Job drawing, mm, ordinate dimensions from the low corner. One solid piece. A direction names the side the tool comes from. Round coordinates to 2 decimals unless told otherwise and drop trailing zeros. Loops run counter-clockwise (first coordinate to the right, second up) from the corner with the lowest first, then second, coordinate; pieces in that order, holes last.
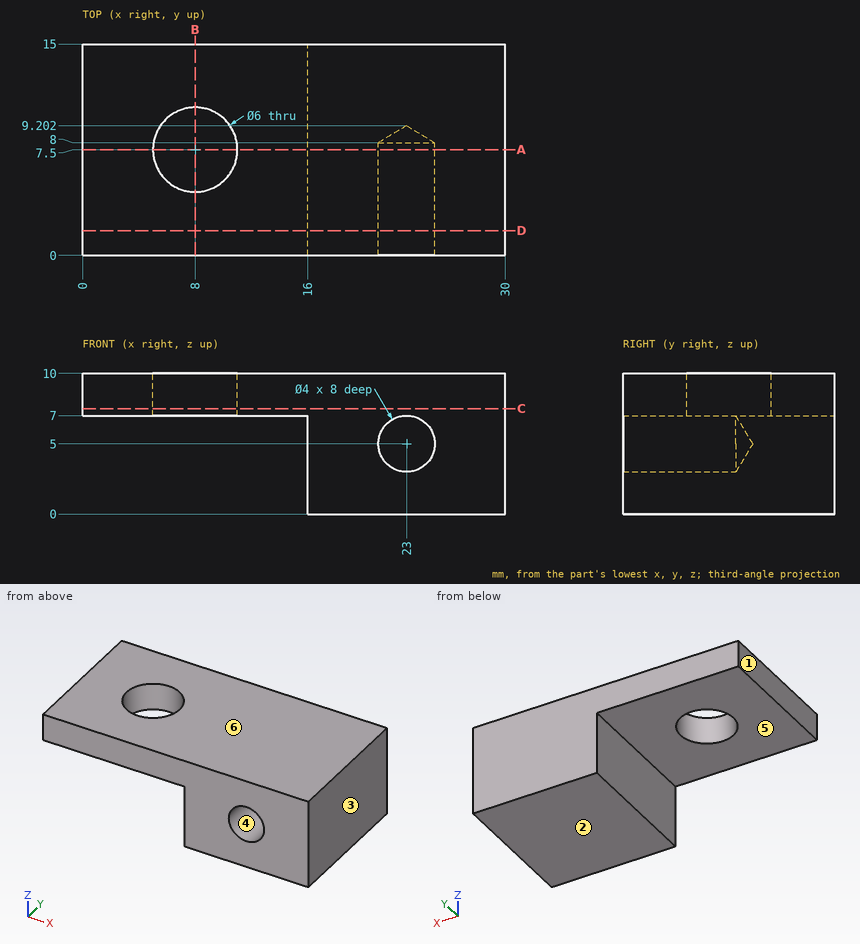
(1) Probe line 1 (Y direction, x = 8, z = 8.1); line 2 (Z direction, x = 23, y = 5.75); line 3 (X direction, y = 6, z = 5). List the from-to ranges inside material, lowest first.
Responses:
line 1: y = 0 to 4.5, 10.5 to 15
line 2: z = 0 to 3, 7 to 10
line 3: x = 16 to 21, 25 to 30
(2) Slice it at A-A on y = 7.5. List the corners of the cut face in (x, z), plus the area to 3 significant figures.
Responses:
outline: (0, 7) - (5, 7) - (5, 10) - (0, 10) - close; (11, 7) - (16, 7) - (16, 0) - (30, 0) - (30, 10) - (11, 10) - close; hole circle Ø4 at (23, 5)
area: 157 mm2
(3) Slice it at C-C on z = 7.5. List the corners of the cut face in (x, y).
Responses:
outline: (0, 0) - (30, 0) - (30, 15) - (0, 15) - close; hole circle Ø6 at (8, 7.5)
(4) Slice it at B-B on x = 8. List the corners of the cut face in (y, z), plus the area to 3 significant figures.
Responses:
outline: (0, 7) - (4.5, 7) - (4.5, 10) - (0, 10) - close; (10.5, 7) - (15, 7) - (15, 10) - (10.5, 10) - close
area: 27.0 mm2
(5) Which spindle directions (+Z, -Z, +X, -X, +Y, -Y) get a long thin tool onto all of the face, cutting with end or side? Do the marked faces 5 and 6. Say none if no direction does.
Responses:
face 5: -Z, -X, +Y, -Y
face 6: +Z, +X, -X, +Y, -Y
(6) Pull direction X, two halves, no side cores. Call the marked faces 1, 2, 3 and 4: +X half, -X half, draft (parallel to the pull), parting line (faces both ways), or undercut.
Responses:
face 1: -X half
face 2: draft
face 3: +X half
face 4: undercut
(7) Pin check, flat tips, straight feed: P1, Ø1.5, axis at x = 3.5, z = 6, coming from the +Y side; P2, Ø1.5, axis at y = 7, z = 3.5, coming from the -X side; P3, Ø4, axis at x = 11.5, z = 6, coming from the -Y side; P4, Ø7.5, axis at x = 6, y = 6, coming from the -Z side. Stop position of each tip, or through.
Responses:
P1: passes through
P2: stops at x = 16
P3: stops at y = 0
P4: stops at z = 7
(8) Slice it at D-D on y = 1.75. List the corners of the cut face in (x, z), plus the area to 3 significant figures.
Responses:
outline: (0, 7) - (16, 7) - (16, 0) - (30, 0) - (30, 10) - (0, 10) - close; hole circle Ø4 at (23, 5)
area: 175 mm2
